CAD build for the part. Positions are in the model's coordinates, mm. Face numbers are marked on the shaded views. A direction names the side the tool comes from. Coordinates: 2 decimals unless noted, no trailing zeros. Write each loop counter-clockwise with the first axis right and the second up, starting at its lowest first coordinate (ties: lowest second). Pieces come first, ordered by that corner, then holes.
```python
from build123d import *

# Parameters (mm, degrees)
SKETCH1_W           = 174.09
SKETCH1_H           = 62.91
SKETCH1_W_2         = 164.29
SKETCH1_H_2         = 53.11
BOSS_EXTRUDE1_DEPTH = 1.6
SKETCH2_W           = 174.09
SKETCH2_H           = 62.91
SKETCH2_W_2         = 152.29
SKETCH2_H_2         = 39.11
BOSS_EXTRUDE2_DEPTH = 3
SKETCH3_W           = 174.09
SKETCH3_H           = 62.91
BOSS_EXTRUDE3_DEPTH = 11.07
SKETCH4_R           = 0.8
CUT_EXTRUDE1_DEPTH  = 10
SKETCH5_R           = 0.75
CUT_EXTRUDE2_DEPTH  = 1.6
FILLET1_R           = 1
SKETCH6_R           = 2
CUT_EXTRUDE3_DEPTH  = 10
CHAMFER1_SIZE       = 1


with BuildPart() as part:
    # Sketch1 → Boss-Extrude1 (new body)
    with BuildSketch(Plane.XY.offset(1006.65)):
        with Locations((-13.164391743, 25.723524096)):
            Rectangle(SKETCH1_W, SKETCH1_H)
        with Locations((-13.164391743, 25.723524096)):
            Rectangle(SKETCH1_W_2, SKETCH1_H_2, mode=Mode.SUBTRACT)
    extrude(amount=-BOSS_EXTRUDE1_DEPTH)

    # Sketch2 → Boss-Extrude2 (add)
    with BuildSketch(Plane.XY.offset(1006.65)):
        with Locations((-13.164391743, 25.723524096)):
            Rectangle(SKETCH2_W, SKETCH2_H)
        with Locations((-13.164391743, 25.723524096)):
            Rectangle(SKETCH2_W_2, SKETCH2_H_2, mode=Mode.SUBTRACT)
    extrude(amount=BOSS_EXTRUDE2_DEPTH)

    # Sketch3 → Boss-Extrude3 (add)
    with BuildSketch(Plane.XY.offset(1009.65)):
        with Locations((-13.164391743, 25.723524096)):
            Rectangle(SKETCH3_W, SKETCH3_H)
        Polygon((61.377029613, 34.213523596), (-87.705813099, 34.213523596), (-88.764391743, 33.154944952), (-88.764391743, 24.613523596), (-88.764391743, 17.57210224), (-87.705813099, 16.513523596), (61.377029613, 16.513523596), (62.435608257, 17.57210224), (62.435608257, 24.613523596), (62.435608257, 33.154944952), align=None, mode=Mode.SUBTRACT)
    extrude(amount=BOSS_EXTRUDE3_DEPTH)

    # Sketch4 → Cut-Extrude1 (cut)
    with BuildSketch(Plane(origin=(0, 0, 1006.65), x_dir=(-1, 0, 0), z_dir=(0, 0, -1))):
        with Locations((-46.835608257, 50.678524096)):
            Circle(SKETCH4_R)
        with Locations((-16.835608257, 50.678524096)):
            Circle(SKETCH4_R)
        with Locations((13.164391743, 50.678524096)):
            Circle(SKETCH4_R)
        with Locations((43.164391743, 50.678524096)):
            Circle(SKETCH4_R)
        with Locations((73.164391743, 50.678524096)):
            Circle(SKETCH4_R)
        with Locations((73.164391743, 0.768524096)):
            Circle(SKETCH4_R)
        with Locations((43.164391743, 0.768524096)):
            Circle(SKETCH4_R)
        with Locations((13.164391743, 0.768524096)):
            Circle(SKETCH4_R)
        with Locations((-16.835608257, 0.768524096)):
            Circle(SKETCH4_R)
        with Locations((-46.835608257, 0.768524096)):
            Circle(SKETCH4_R)
    extrude(amount=-CUT_EXTRUDE1_DEPTH, mode=Mode.SUBTRACT)

    # Sketch5 → Cut-Extrude2 (cut)
    with BuildSketch(Plane(origin=(0, 0, 1005.05), x_dir=(-1, 0, 0), z_dir=(0, 0, -1))):
        with Locations((95.309391743, 52.278524096)):
            Circle(SKETCH5_R)
        with Locations((95.309391743, -0.831475904)):
            Circle(SKETCH5_R)
        with Locations((-68.980608257, -0.831475904)):
            Circle(SKETCH5_R)
        with Locations((-68.980608257, 52.278524096)):
            Circle(SKETCH5_R)
    extrude(amount=-CUT_EXTRUDE2_DEPTH, mode=Mode.SUBTRACT)

    # Fillet1
    fillet1_edges = [part.edges().sort_by_distance(p)[0] for p in [
        (68.980608257, 51.528524096, 1005.85),
        (68.230608257, 52.278524096, 1005.85),
        (68.230608257, -0.831475904, 1005.85),
        (68.980608257, -0.081475904, 1005.85),
        (-95.309391743, -0.081475904, 1005.85),
        (-94.559391743, -0.831475904, 1005.85),
        (-95.309391743, 51.528524096, 1005.85),
        (-94.559391743, 52.278524096, 1005.85),
    ]]
    fillet(fillet1_edges, radius=FILLET1_R)

    # Sketch6 → Cut-Extrude3 (cut)
    with BuildSketch(Plane.XY.offset(1020.72)):
        with Locations((-93.164391743, 38.613523596)):
            Circle(SKETCH6_R)
        with Locations((-53.164391743, 38.613523596)):
            Circle(SKETCH6_R)
        with Locations((-13.164391743, 38.613523596)):
            Circle(SKETCH6_R)
        with Locations((26.835608257, 38.613523596)):
            Circle(SKETCH6_R)
        with Locations((66.835608257, 38.613523596)):
            Circle(SKETCH6_R)
        with Locations((66.835608257, 12.113523596)):
            Circle(SKETCH6_R)
        with Locations((26.835608257, 12.113523596)):
            Circle(SKETCH6_R)
        with Locations((-13.164391743, 12.113523596)):
            Circle(SKETCH6_R)
        with Locations((-53.164391743, 12.113523596)):
            Circle(SKETCH6_R)
        with Locations((-93.164391743, 12.113523596)):
            Circle(SKETCH6_R)
    extrude(amount=-CUT_EXTRUDE3_DEPTH, mode=Mode.SUBTRACT)

    # Chamfer1
    chamfer1_edges = [part.edges().sort_by_distance(p)[0] for p in [
        (73.880608257, 57.178524096, 1012.885),
        (73.880608257, -5.731475904, 1012.885),
        (-100.209391743, -5.731475904, 1012.885),
        (-100.209391743, 57.178524096, 1012.885),
        (-13.164391743, 57.178524096, 1020.72),
        (-100.209391743, 25.723524096, 1020.72),
        (-13.164391743, -5.731475904, 1020.72),
        (73.880608257, 25.723524096, 1020.72),
        (-100.209391743, 25.723524096, 1005.05),
    ]]
    chamfer(chamfer1_edges, length=CHAMFER1_SIZE)


solid = part.part
```
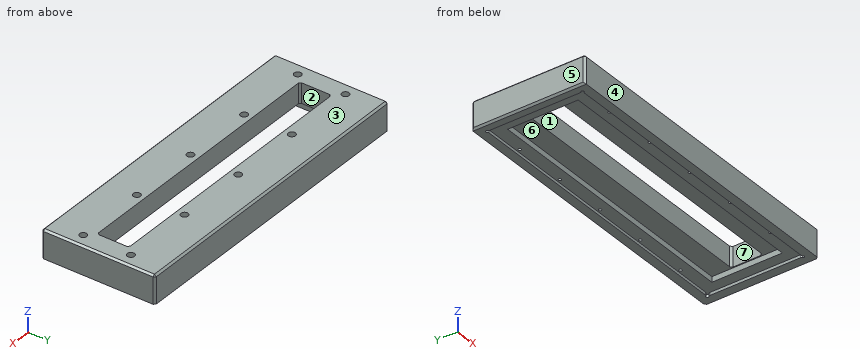
Item 1: Saw through at D-D, the plane z = 1014.25. State how many separate pieces and enclosed holes the cut face has, and give its area (3 significant figures).
Item 2: Saw through at B-B, the plane x = -22.5. Write the cut outline in (y, z), and give its area (3 significant figures).
Item 3: Two-plate mould, pull along Y, no slides. Class the marked faces 1, 2, 3 and 4: +Y half, -Y half, draft (parallel to the pull), parting line (faces both ways), or undercut.
Item 4: Saw through at C-C, the plane y = 31. Write the cut outline in (x, z).
Item 5: Flat gauge pins, fed straight in: pin 1 Ø1.3 at (x, y) = (-43, 1) entering from -Z; pin 2 Ø4 at (x, y) = (46, 14.5) entering from -Z; pin 3 Ø0.8 at (x, y) = (17, 0.5) entering from -Z. Where does each tip first touch, or does it go through?
Item 6: Saw through at A-A, the plane y = 47. Write the cut outline in (x, z).
Item 7: Wall check: line 1 along X through (y, z) = (23.5, 1011); line 2 along X through (y, z) = (14, 1008.75); line 3 along Y through (x, z) = (-19, 1009). Give the ranges that are in metal, low to high.
Item 8: Which spindle directions (+Z, -Z, +X, -X, +Y, -Y) get a long thin tool onto all of the face, cutting with end or side? Do the marked faces 5, 6 and 7. Say none if no direction does.
Working result:
1. separate pieces: 1
1. enclosed holes: 21
1. area: 8,130 mm2
2. outline: (-5.73, 1005.05) - (-0.83, 1005.05) - (-0.83, 1006.65) - (6.17, 1006.65) - (6.17, 1009.65) - (16.51, 1009.65) - (16.51, 1020.72) - (-4.73, 1020.72) - (-5.73, 1019.72) - close; (34.21, 1009.65) - (45.28, 1009.65) - (45.28, 1006.65) - (52.28, 1006.65) - (52.28, 1005.05) - (57.18, 1005.05) - (57.18, 1019.72) - (56.18, 1020.72) - (34.21, 1020.72) - close
2. area: 587 mm2
3. face 1: undercut
3. face 2: undercut
3. face 3: draft
3. face 4: -Y half
4. outline: (-100.21, 1006.05) - (-99.21, 1005.05) - (-95.31, 1005.05) - (-95.31, 1006.65) - (-89.31, 1006.65) - (-89.31, 1009.65) - (-88.76, 1009.65) - (-88.76, 1020.72) - (-99.21, 1020.72) - (-100.21, 1019.72) - close; (62.44, 1009.65) - (62.98, 1009.65) - (62.98, 1006.65) - (68.98, 1006.65) - (68.98, 1005.05) - (73.88, 1005.05) - (73.88, 1019.72) - (72.88, 1020.72) - (62.44, 1020.72) - close
5. pin 1: stops at z = 1006.65
5. pin 2: stops at z = 1009.65
5. pin 3: stops at z = 1016.65
6. outline: (-100.21, 1006.05) - (-99.21, 1005.05) - (-95.31, 1005.05) - (-95.31, 1006.65) - (68.98, 1006.65) - (68.98, 1005.05) - (73.88, 1005.05) - (73.88, 1019.72) - (72.88, 1020.72) - (-99.21, 1020.72) - (-100.21, 1019.72) - close
7. line 1: x = -100.21 to -88.76, 62.44 to 73.88
7. line 2: x = -100.21 to -89.31, 62.98 to 73.88
7. line 3: y = -5.73 to 6.17, 45.28 to 57.18
8. face 5: +Z, -Z, -X, +Y, -Y
8. face 6: -Z
8. face 7: +Z, -Z
